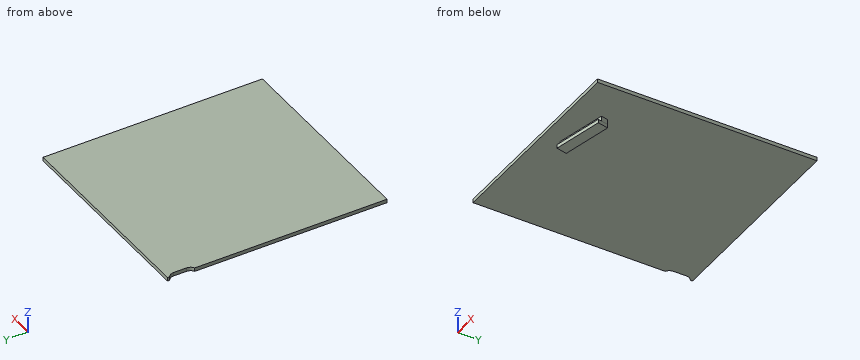
```python
from build123d import *

# Parameters (mm, degrees)
SKETCH1_W           = 280
SKETCH1_H           = 300
BOSS_EXTRUDE1_DEPTH = 5
CUT_EXTRUDE1_DEPTH  = 6
BOSS_EXTRUDE2_DEPTH = 7
BOSS_EXTRUDE3_DEPTH = 5


with BuildPart() as part:
    # Sketch1 → Boss-Extrude1 (new body)
    with BuildSketch(Plane.XY):
        Rectangle(SKETCH1_W, SKETCH1_H)
    extrude(amount=BOSS_EXTRUDE1_DEPTH)

    # Sketch2 → Cut-Extrude1 (cut, through all)
    with BuildSketch(Plane.XY.offset(5)):
        with BuildLine():
            Line((-153, 139), (-153, 121))
            ThreePointArc((-153, 121), (-144, 112), (-135, 121))
            Line((-135, 121), (-135, 139))
            ThreePointArc((-135, 139), (-144, 148), (-153, 139))
        make_face()
    extrude(amount=-CUT_EXTRUDE1_DEPTH, mode=Mode.SUBTRACT)

    # Sketch3 → Boss-Extrude2 (add)
    with BuildSketch(Plane(origin=(0, 0, 0), x_dir=(-1, 0, 0), z_dir=(0, 0, -1))):
        Polygon((-82.857142857, -101.5), (-14.483171201, -116.5), (-16.626028344, -126.267710237), (-85, -111.267710237), align=None)
    extrude(amount=BOSS_EXTRUDE2_DEPTH)

    # Sketch4 → Boss-Extrude3 (add)
    with BuildSketch(Plane(origin=(0, 0, -7), x_dir=(-1, 0, 0), z_dir=(0, 0, -1))):
        Polygon((-82.857142857, -101.5), (-14.483171201, -116.5), (-17.697456916, -131.151565355), (-86.071428571, -116.151565355), align=None)
    extrude(amount=BOSS_EXTRUDE3_DEPTH)


solid = part.part
```
Model file for the job. Use its own axes, mm. Coordinates: 2 decimals unless noted, no trailing zeros. Order: outer loops, then holes, each group sorted by start corner. A loop starts at its lowest first (then second) coordinate and runs counter-clockwise, first axis right, second up. Notation, with made-up numbers: (80.5, 86.5) - (84.5, 86.5) arc R22 cw to (84.5, 108.5) - close; hole circle Ø9 at (37.5, -16). An arc over 180 degrees is marked (long way). Return JSON: item names as keys, results as strings. Group by question number.
1) Saw through at B-B, the plane x = -33. Write the cut outline in (y, z), plus the area to 3 significant figures.
2) Saw through at A-A, the plane y = -107. Write the cut outline in (x, z).
3) Saw through at D-D, the plane x = 59. Write the cut outline in (y, z), plus the area to 3 significant figures.
4) Saw through at C-C, the plane y = -15. Write the cut outline in (x, z), plus the area to 3 significant figures.
5) Probe line 1 (Z direction, x = 110.5, y = 18); line 2 (X direction, y = 136, z = 1.75); line 3 (Y direction, x = 34.5, z = -0.75). List the from-to ranges inside material, lowest first. Write a range as from..to.
6) Flat gauge pins, fed straight in: P1, Ø1, axis at x = 61, z = -9.5, coming from the +Y side; P2, Ø5, axis at x = 106.5, y = -9.5, coming from the -Z side; P3, Ø8, axis at y = 79, z = -1, coming from the -X side; P4, Ø5.5, axis at y = 134, z = 2, coming from the -X side. Where does each tip first touch, or does it go through?
Values found:
{
 "1": {"outline": "(-150, 0) - (150, 0) - (150, 5) - (-150, 5) - close", "area": "1,500 mm²"},
 "2": {"outline": "(-140, 0) - (57.79, 0) - (57.79, -12) - (84.06, -12) - (84.06, 0) - (140, 0) - (140, 5) - (-140, 5) - close"},
 "3": {"outline": "(-150, 0) - (-116.97, 0) - (-116.97, -7) - (-122.09, -7) - (-122.09, -12) - (-106.73, -12) - (-106.73, 0) - (150, 0) - (150, 5) - (-150, 5) - close", "area": "1,650 mm²"},
 "4": {"outline": "(-140, 0) - (140, 0) - (140, 5) - (-140, 5) - close", "area": "1,400 mm²"},
 "5": {"line 1": "z = 0..5", "line 2": "x = -135..140", "line 3": "y = -122.35..-112.11"},
 "6": {"P1": "stops at y = -106.19", "P2": "stops at z = 0", "P3": "stops at x = -140", "P4": "stops at x = -135"}
}
